Here's how the part is built. I have some questions about the finished solid (model axes, mm). Round coordinates to 2 decimals unless told otherwise and drop trailing zeros. Loops run counter-clockwise (first coordinate to the right, second up) from the corner with the lowest first, then second, coordinate; pieces in that order, holes last. Notation, with made-up numbers: M -7,-21 L 19,-21 A29 ccw 19,12 Z; hole C -1,25 d4. An arc over 180 degrees is marked long. Answer as a JSON object with one key per item and string values.
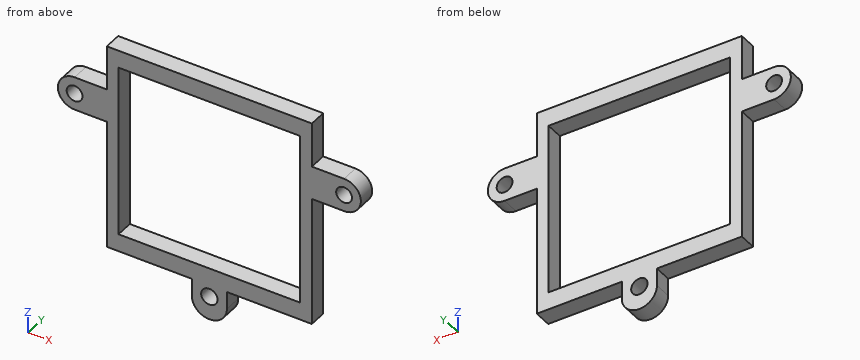
from build123d import *

# Parameters (mm, degrees)
SKETCH1_R           = 1.35
SKETCH1_W           = 35
SKETCH1_H           = 35.5
SKETCH1_W_2         = 31
SKETCH1_H_2         = 29.5
SKETCH1_R_2         = 1.4
BOSS_EXTRUDE3_DEPTH = 3


with BuildPart() as part:
    # Sketch1 → Boss-Extrude3 (new body)
    # profile 1 of 4: a face of its own
    with BuildSketch(Plane(origin=(0, 0, 0), x_dir=(1, 0, 0), z_dir=(0, 1, 0))):
        with BuildLine():
            Line((-17.5, -10.110115741), (-17.5, -4.389884259))
            Line((-17.5, -4.389884259), (-23, -4.389884259))
            ThreePointArc((-23, -4.389884259), (-25.860115741, -7.25), (-23, -10.110115741))
            Line((-23, -10.110115741), (-17.5, -10.110115741))
        make_face()
        with Locations(Location((-23, -7.25, 0), (0, 0, 270))):
            Circle(SKETCH1_R, mode=Mode.SUBTRACT)
    # profile 2 of 4: a face of its own
    with BuildSketch(Plane(origin=(0, 0, 0), x_dir=(1, 0, 0), z_dir=(0, 1, 0))):
        Rectangle(SKETCH1_W, SKETCH1_H)
        Rectangle(SKETCH1_W_2, SKETCH1_H_2, mode=Mode.SUBTRACT)
    # profile 3 of 4: a face of its own
    with BuildSketch(Plane(origin=(0, 0, 0), x_dir=(1, 0, 0), z_dir=(0, 1, 0))):
        with BuildLine():
            Line((23, -4.389884259), (17.5, -4.389884259))
            Line((17.5, -4.389884259), (17.5, -10.110115741))
            Line((17.5, -10.110115741), (23, -10.110115741))
            ThreePointArc((23, -10.110115741), (25.860115741, -7.25), (23, -4.389884259))
        make_face()
        with Locations(Location((23, -7.25, 0), (0, 0, 270))):
            Circle(SKETCH1_R, mode=Mode.SUBTRACT)
    # profile 4 of 4: a face of its own
    with BuildSketch(Plane(origin=(0, 0, 0), x_dir=(1, 0, 0), z_dir=(0, 1, 0))):
        with BuildLine():
            Line((-3, 20.75), (-3, 17.75))
            Line((-3, 17.75), (3, 17.75))
            Line((3, 17.75), (3, 20.75))
            ThreePointArc((3, 20.75), (0, 23.75), (-3, 20.75))
        make_face()
        with Locations(Location((0, 19.75, 0), (0, 0, 270))):
            Circle(SKETCH1_R_2, mode=Mode.SUBTRACT)
    extrude(amount=BOSS_EXTRUDE3_DEPTH)


solid = part.part
Item 1: Please list where these lines run through material, in increasing order: probe 1 along X at (y, z) = (2.05, 7.25); probe 2 along X at (y, z) = (0.45, 1); probe 3 along X at (y, z) = (0.7, -19.75). Write a range as from..to.
Resolved:
{"probe 1": "-25.86..-24.35, -21.65..-15.5, 15.5..21.65, 24.35..25.86", "probe 2": "-17.5..-15.5, 15.5..17.5", "probe 3": "-3..-1.4, 1.4..3"}
Item 2: I want a section at C-C, the plane z = 7.25. Please give me the cut outline in (x, y), then the cut area to 3 significant figures.
Resolved:
{"outline": "M -25.86,0 L -24.35,0 L -24.35,3 L -25.86,3 Z; M -21.65,0 L -15.5,0 L -15.5,3 L -21.65,3 Z; M 15.5,0 L 21.65,0 L 21.65,3 L 15.5,3 Z; M 24.35,0 L 25.86,0 L 25.86,3 L 24.35,3 Z", "area": "46.0 mm²"}
Item 3: I want a section at D-D, the plane y = 1.85. Please give me the cut outline in (x, z), then the cut area to 3 significant figures.
Resolved:
{"outline": "M -23,4.39 L -17.5,4.39 L -17.5,-17.75 L -3,-17.75 L -3,-20.75 A3 ccw 3,-20.75 L 3,-17.75 L 17.5,-17.75 L 17.5,4.39 L 23,4.39 A2.86 ccw 23,10.11 L 17.5,10.11 L 17.5,17.75 L -17.5,17.75 L -17.5,10.11 L -23,10.11 A2.86 ccw Z; hole C -23,7.25 d2.7; hole M -15.5,-14.75 L 15.5,-14.75 L 15.5,14.75 L -15.5,14.75 Z; hole C 0,-19.75 d2.8; hole C 23,7.25 d2.7", "area": "431 mm²"}
Item 4: I'm going to push flat-ended pins straight in: pin 1 Ø0.9 at (x, y) = (21.5, 1.5) entering from +Z; pin 2 Ø1.5 at (y, z) = (1, 13) entering from +X; pin 3 Ø0.9 at (y, z) = (2, 1) entering from -X. Where does each tip first touch, or does it pass through?
Resolved:
{"pin 1": "z = 10.11", "pin 2": "x = 17.5", "pin 3": "x = -17.5"}
Item 5: I want a section at B-B, the plane x = 0. Please give me the cut outline in (y, z).
Resolved:
{"outline": "M 0,-23.75 L 3,-23.75 L 3,-21.15 L 0,-21.15 Z; M 0,-18.35 L 3,-18.35 L 3,-14.75 L 0,-14.75 Z; M 0,14.75 L 3,14.75 L 3,17.75 L 0,17.75 Z"}
Item 6: I want a section at A-A, the plane z = -9. Please give me the cut outline in (x, y), then the cut area to 3 significant figures.
Resolved:
{"outline": "M -17.5,0 L -15.5,0 L -15.5,3 L -17.5,3 Z; M 15.5,0 L 17.5,0 L 17.5,3 L 15.5,3 Z", "area": "12.0 mm²"}
